```python
from build123d import *

# Parameters (mm, degrees)
BOSS_EXTRUDE1_DEPTH = 21.8


with BuildPart() as part:
    # Sketch1 → Boss-Extrude1 (new body)
    with BuildSketch(Plane.XY):
        with BuildLine():
            Line((239.323919844, -47.477038572), (231.477637601, -45.916315996))
            ThreePointArc((231.477637601, -45.916315996), (236, 0), (231.477637601, 45.916315996))
            Line((231.477637601, 45.916315996), (239.323919844, 47.477038572))
            ThreePointArc((239.323919844, 47.477038572), (244, 0), (239.323919844, -47.477038572))
        make_face()
        Polygon((236.510641242, 27.859172504), (234.226095505, 30.836450473), (235.662220993, 34.303564103), (239.382892217, 34.793399762), (241.667437954, 31.816121792), (240.231312467, 28.349008163), align=None, mode=Mode.SUBTRACT)
        Polygon((241.876388375, -3.25), (243.75277675, 0), (241.876388375, 3.25), (238.123611625, 3.25), (236.24722325, 0), (238.123611625, -3.25), align=None, mode=Mode.SUBTRACT)
        Polygon((235.662220993, -34.303564103), (239.382892217, -34.793399762), (241.667437954, -31.816121792), (240.231312467, -28.349008163), (236.510641242, -27.859172504), (234.226095505, -30.836450473), align=None, mode=Mode.SUBTRACT)
    extrude(amount=BOSS_EXTRUDE1_DEPTH)


solid = part.part
```
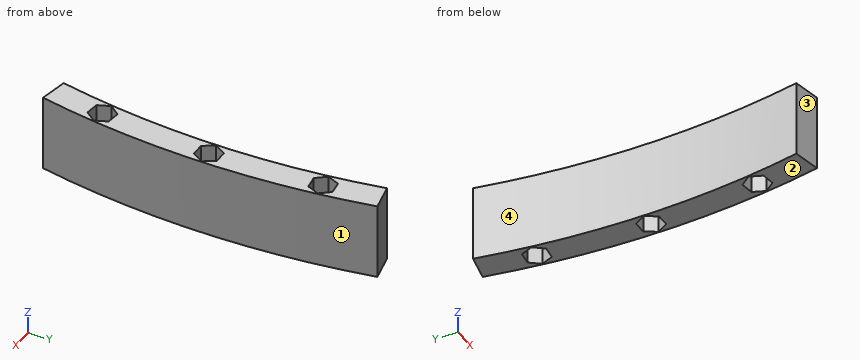
Design review of the part built by this model. Coordinates are the model's own, in mm. Face numbers are marked on the shaded views. Give positions to 0.01 mm unless a question says otherwise; leave off trailing zeros. Loops run counter-clockwise (first coordinate to the right, second up) from the corner with the lowest first, then second, coordinate; pieces in that order, holes last. Notation, with made-up numbers: (79.5, 16.5) -> (113.5, 16.5) arc R19 cw to (113.5, 53.5) -> close; hole circle Ø2 at (-0.75, 22). An arc over 180 degrees is marked (long way). One line per item, written item: value.
Q1. Draft analysis for pull direction Y (two halves, no side actions). For the marked faces 1, 2, 3 and 4, state which applies: pulls with the +Y half, pulls with the -Y half, needs draft (parallel to the pull), parting line crosses it, or undercut.
Numbers:
face 1: parting line crosses it
face 2: needs draft
face 3: pulls with the -Y half
face 4: undercut
Q2. For pin 1 Ø1.9 at (x, z) = (239.5, 9.5) entering from -Y; pin 2 Ø1 at (x, z) = (234, 17) entering from +Y; pin 3 Ø6 at (x, z) = (239, 14.5) entering from +Y, all flat-tipped, find the tip position at first contact; note any pin that passes through.
Numbers:
pin 1: stops at y = -47.48
pin 2: stops at y = 46.52
pin 3: stops at y = 47.48
Q3. We need section B-B on y = 33.5. Give the boundary of the cut face in (x, z), and give its area (3 significant figures).
Numbers:
outline: (233.6, 0) -> (235.33, 0) -> (235.33, 21.8) -> (233.6, 21.8) -> close; (240.38, 0) -> (241.68, 0) -> (241.68, 21.8) -> (240.38, 21.8) -> close
area: 66.1 mm^2
Q4. We need section D-D on y = 12. Give the boundary of the cut face in (x, z).
Numbers:
outline: (235.69, 0) -> (243.7, 0) -> (243.7, 21.8) -> (235.69, 21.8) -> close
Q5. We need section C-C on y = -37.5. Give the boundary of the cut face in (x, z), and give its area (3 significant figures).
Numbers:
outline: (232.99, 0) -> (241.09, 0) -> (241.09, 21.8) -> (232.99, 21.8) -> close
area: 177 mm^2
Q6. For L1, parallel to Y at x = 238.75, z = 7.25; L2, parallel to Y at x = 238.5, z = 19.25; L3, parallel to X at y = 1.5, z = 11, list the stretches that pass through material, from the lowest coordinate up.
Numbers:
L1: y = -47.36 to -34.71, -28.15 to -3.25, 3.25 to 28.15, 34.71 to 47.36
L2: y = -47.31 to -34.68, -28.12 to -3.25, 3.25 to 28.12, 34.68 to 47.31
L3: x = 236 to 237.11, 242.89 to 244
Q7. We need section A-A on z = 13.5. Give the boundary of the cut face in (x, y).
Numbers:
outline: (231.48, -45.92) -> (239.32, -47.48) arc R243.36 ccw to (239.32, 47.48) -> (231.48, 45.92) arc R235.36 cw to start; hole (234.23, -30.84) -> (235.66, -34.3) -> (239.38, -34.79) -> (241.67, -31.82) -> (240.23, -28.35) -> (236.51, -27.86) -> close; hole (234.23, 30.84) -> (236.51, 27.86) -> (240.23, 28.35) -> (241.67, 31.82) -> (239.38, 34.79) -> (235.66, 34.3) -> close; hole (236.25, 0) -> (238.12, -3.25) -> (241.88, -3.25) -> (243.75, 0) -> (241.88, 3.25) -> (238.12, 3.25) -> close
